```python
from build123d import *

# Parameters (mm, degrees)
BOSS_EXTRUDE1_DEPTH     = 3.175
SKETCH2_R               = 6.35
CUT_EXTRUDE1_DEPTH      = 4.1750001
CUT_EXTRUDE2_DEPTH      = 13.851031146
CUT_EXTRUDE2_DEPTH_BACK = 13.851031146


with BuildPart() as part:
    # Sketch1 → Boss-Extrude1 (new body)
    with BuildSketch(Plane.XY):
        with BuildLine():
            add(Edge.make_bspline(
                [(214.122, 0.26979372), (214.042517561, 0.336401081), (213.528971009, 0.273510814), (212.614475706, 0.530942112), (210.937412976, 0.69005818), (208.678154781, 1.031540783), (205.767891794, 1.412612557), (202.258298365, 1.882266), (198.158505405, 2.4131646), (193.498201346, 3.004251359), (188.3046229, 3.645171414), (182.610259265, 4.327250831), (176.450111776, 5.042029836), (169.862114854, 5.779776892), (162.886908752, 6.531484704), (155.567547263, 7.287816965), (147.949138879, 8.039011284), (140.078674392, 8.774523149), (132.004623532, 9.484696808), (123.776853773, 10.157659428), (115.445921162, 10.782438327), (107.063264355, 11.347433986), (98.680532246, 11.840832833), (90.349330839, 12.250169768), (82.121113367, 12.564529441), (74.046372156, 12.77365626), (66.175007458, 12.867335678), (58.555385553, 12.838133258), (51.234483397, 12.680408315), (44.257364483, 12.390162696), (37.666974317, 11.966637162), (31.503817676, 11.411106073), (25.805608692, 10.727908153), (20.607079774, 9.922856403), (15.939732749, 9.004358901), (11.830923582, 7.982801344), (8.304000309, 6.868145192), (5.376882013, 5.670771919), (3.058903356, 4.398782317), (1.353631156, 3.049665872), (0.261418186, 1.590784391), (-0.121830169, 0), (0.261418186, -1.590784391), (1.353631156, -3.049665872), (3.058903356, -4.398782317), (5.376882013, -5.670771919), (8.304000309, -6.868145192), (11.830923582, -7.982801344), (15.939732749, -9.004358901), (20.607079774, -9.922856403), (25.805608692, -10.727908153), (31.503817676, -11.411106073), (37.666974317, -11.966637162), (44.257364483, -12.390162696), (51.234483397, -12.680408315), (58.555385553, -12.838133258), (66.175007458, -12.867335678), (74.046372156, -12.77365626), (82.121113367, -12.564529441), (90.349330839, -12.250169768), (98.680532246, -11.840832833), (107.063264355, -11.347433986), (115.445921162, -10.782438327), (123.776853773, -10.157659428), (132.004623532, -9.484696808), (140.078674392, -8.774523149), (147.949138879, -8.039011284), (155.567547263, -7.287816965), (162.886908752, -6.531484704), (169.862114854, -5.779776892), (176.450111776, -5.042029836), (182.610259265, -4.327250831), (188.3046229, -3.645171414), (193.498201346, -3.004251359), (198.158505405, -2.4131646), (202.258298365, -1.882266), (205.767891794, -1.412612557), (208.678154781, -1.031540783), (210.937412976, -0.69005818), (212.614475706, -0.530942112), (213.528971009, -0.273510814), (214.25071943, -0.361898032), (214.25071943, 0.161925093), (214.122, 0.26979372)],
                knots=[0, 0, 0, 0, 0.000762215, 0.003044706, 0.006832246, 0.012101176, 0.018817536, 0.026939455, 0.036414848, 0.047184629, 0.059180413, 0.072327874, 0.086544061, 0.10174058, 0.117823336, 0.134691452, 0.152240154, 0.17036129, 0.188941008, 0.207865435, 0.227016078, 0.246275696, 0.265524943, 0.284644966, 0.303520118, 0.322034575, 0.340078353, 0.357542593, 0.374325482, 0.390329891, 0.40546389, 0.419643801, 0.432793371, 0.444843817, 0.455737921, 0.465428653, 0.47388632, 0.481101634, 0.487101684, 0.491975368, 0.495930678, 0.499382808, 0.502834938, 0.506790248, 0.511663932, 0.517663982, 0.524879296, 0.533336963, 0.543027695, 0.553921799, 0.565972245, 0.579121815, 0.593301726, 0.608435725, 0.624440134, 0.641223023, 0.658687263, 0.676731041, 0.695245498, 0.71412065, 0.733240673, 0.75248992, 0.771749538, 0.790900181, 0.809824608, 0.828404326, 0.846525462, 0.864074164, 0.88094228, 0.897025036, 0.912221555, 0.926437743, 0.939585203, 0.951580988, 0.962350768, 0.971826161, 0.979948081, 0.98666444, 0.991933371, 0.99572091, 0.998003402, 0.998765616, 1, 1, 1, 1], degree=3))
        make_face()
    extrude(amount=BOSS_EXTRUDE1_DEPTH)

    # Sketch2 → Cut-Extrude1 (cut, through all)
    with BuildSketch(Plane.XY.offset(3.175)):
        with Locations((25.4, 0)):
            Circle(SKETCH2_R)
        with Locations((101.6, 0)):
            Circle(SKETCH2_R)
    extrude(amount=-CUT_EXTRUDE1_DEPTH, mode=Mode.SUBTRACT)

    # Sketch4 → Cut-Extrude2 (cut, two sides)
    with BuildSketch(Plane(origin=(0, 0, 0), x_dir=(1, 0, 0), z_dir=(0, 1, 0))) as cut_extrude2_sk:
        Polygon((131.301372669, 0), (130.854723983, -3.175), (214.218539573, -3.175), (214.218539573, 0), align=None)
    extrude(amount=CUT_EXTRUDE2_DEPTH, mode=Mode.SUBTRACT)
    extrude(cut_extrude2_sk.sketch, amount=-CUT_EXTRUDE2_DEPTH_BACK, mode=Mode.SUBTRACT)

    # Sketch6 → Cut-Loft1 section 0
    with BuildSketch(Plane.XY.offset(3.175)):
        with BuildLine():
            Line((19.05, -5.856388973), (19.05, -9.60451625))
            Line((19.05, -9.60451625), (19.05, -13.496705478))
            Line((19.05, -13.496705478), (-3.17679028, -18.7418168))
            Line((-3.17679028, -18.7418168), (-7.400210772, 8.670878009))
            Line((-7.400210772, 8.670878009), (19.05, 13.499844305))
            Line((19.05, 13.499844305), (19.05, 9.60451625))
            Line((19.05, 9.60451625), (19.05, 5.856388972))
            Line((19.05, 5.856388972), (16.002, 5.855689085))
            add(Edge.make_bspline(
                [(16.002, 5.855689085), (15.278985699, 5.689672728), (14.191834186, 5.424851558), (12.757843363, 5.037907465), (11.69367278, 4.729775055), (10.646700316, 4.403337894), (9.617692504, 4.055796047), (8.608301637, 3.684577658), (7.626216232, 3.28790719), (6.678573411, 2.8637313), (5.779182107, 2.40890834), (5.078910801, 2.000461241), (4.5709467, 1.665455737), (4.220151013, 1.411514439), (3.905914023, 1.157647081), (3.631157505, 0.904651906), (3.399885574, 0.653944439), (3.226743451, 0.433066972), (3.126676284, 0.2697322), (3.07552602, 0.144421915), (3.049218429, 0.037663177), (3.047390298, 5.5e-08), (3.04921854, -0.03766331), (3.075525744, -0.1444217), (3.126676947, -0.269732641), (3.226742145, -0.433066135), (3.399888053, -0.653946015), (3.631152817, -0.904648933), (3.905923107, -1.157652839), (4.220131475, -1.411502059), (4.570981553, -1.665477812), (5.078773369, -2.000374258), (5.77925724, -2.408956031), (6.678536824, -2.863707828), (7.626233895, -3.287919031), (8.608295197, -3.684572243), (9.617690306, -4.05579733), (10.64671253, -4.403340225), (11.693641898, -4.729767367), (12.757897505, -5.037921267), (14.191640812, -5.424801637), (15.278985699, -5.689672728), (16.002, -5.855689085)],
                knots=[0, 0, 0, 0, 0.0625, 0.09375, 0.125, 0.15625, 0.1875, 0.21875, 0.25, 0.28125, 0.3125, 0.34375, 0.359375, 0.375, 0.390625, 0.40625, 0.421875, 0.4375, 0.453125, 0.46875, 0.484375, 0.5, 0.515625, 0.53125, 0.546875, 0.5625, 0.578125, 0.59375, 0.609375, 0.625, 0.640625, 0.65625, 0.6875, 0.71875, 0.75, 0.78125, 0.8125, 0.84375, 0.875, 0.90625, 0.9375, 1, 1, 1, 1], degree=3))
            Line((16.002, -5.855689085), (19.05, -5.856388973))
        make_face()
    # Sketch5 → Cut-Loft1 section 1
    with BuildSketch(Plane(origin=(0, 0, 0), x_dir=(-1, 0, 0), z_dir=(0, 0, -1))):
        with BuildLine():
            Line((-19.05, -9.69489598), (-19.05, -5.952242124))
            Line((-19.05, -5.952242124), (-16.002, -5.952242124))
            add(Edge.make_bspline(
                [(-16.002, 5.952242124), (-15.254770655, 5.78657596), (-14.131320952, 5.521981031), (-12.64893123, 5.134599211), (-11.548436123, 4.825723352), (-10.465051878, 4.498073941), (-9.399590771, 4.148800211), (-8.353696965, 3.775270971), (-7.504851445, 3.442218555), (-6.842934482, 3.161623807), (-6.194794877, 2.871042337), (-5.414728041, 2.488039147), (-4.683877816, 2.074629942), (-4.151373193, 1.734752799), (-3.782164679, 1.476616997), (-3.449549124, 1.21792525), (-3.156545696, 0.959314296), (-2.90735717, 0.702084345), (-2.716911913, 0.473376027), (-2.620007494, 0.329250424), (-2.568278365, 0.232230216), (-2.539730887, 0.166366119), (-2.518563335, 0.105023254), (-2.505407276, 0.055343345), (-2.499698937, 0.022962059), (-2.498722808, 3.7e-08), (-2.499699014, -0.022962102), (-2.505407277, -0.055343359), (-2.518563346, -0.105023288), (-2.539730598, -0.166365891), (-2.568278462, -0.232230258), (-2.620012631, -0.329254292), (-2.716907842, -0.47337309), (-2.907361053, -0.702086989), (-3.156540251, -0.959310743), (-3.449558648, -1.217931354), (-3.782145051, -1.476604524), (-4.151407833, -1.734774759), (-4.683741695, -2.074543768), (-5.414804155, -2.48808676), (-6.194777113, -2.871030834), (-6.84292503, -3.16161805), (-7.50486635, -3.442227642), (-8.353689563, -3.77526546), (-9.399589141, -4.148801556), (-10.465063669, -4.498076208), (-11.54840573, -4.825715767), (-12.648984703, -5.134612855), (-14.131129756, -5.52193166), (-15.254770655, -5.78657596), (-16.002, -5.952242124)],
                knots=[0, 0, 0, 0, 0.0625, 0.09375, 0.125, 0.15625, 0.1875, 0.21875, 0.25, 0.265625, 0.28125, 0.3125, 0.34375, 0.359375, 0.375, 0.390625, 0.40625, 0.421875, 0.4375, 0.453125, 0.4609375, 0.46875, 0.4765625, 0.484375, 0.4921875, 0.5, 0.5078125, 0.515625, 0.5234375, 0.53125, 0.5390625, 0.546875, 0.5625, 0.578125, 0.59375, 0.609375, 0.625, 0.640625, 0.65625, 0.6875, 0.71875, 0.734375, 0.75, 0.78125, 0.8125, 0.84375, 0.875, 0.90625, 0.9375, 1, 1, 1, 1], degree=3))
            Line((-16.002, 5.952242124), (-19.05, 5.952242124))
            Line((-19.05, 5.952242124), (-19.05, 9.69489598))
            Line((-19.05, 9.69489598), (-19.05, 12.377646409))
            Line((-19.05, 12.377646409), (3.93721866, 8.635694366))
            Line((3.93721866, 8.635694366), (2.51171312, -11.744580154))
            Line((2.51171312, -11.744580154), (-19.05, -12.301418255))
            Line((-19.05, -12.301418255), (-19.05, -9.69489598))
        make_face()
    loft(mode=Mode.SUBTRACT)


solid = part.part
```
Could you check a few things on this model? Use its own coordinates, in mm. Give positions to 0.01 mm unless a question says otherwise; leave off trailing zeros. One line per item, written item: value. Start each with the question number.
Item 1: Imagine slicing it at A-A, the plane y = 0. Give the number of separate pieces and of enclosed holes in the cut face, and give its area (3 significant figures).
Item 2: I'm going to push flat-ended pins straight in: pin 1 (10 mm diameter, centred on x = 25.4, y = 0, fed in from +Z); pin 2 (12 mm diameter, centred on x = 77, y = -8, fed in from -Z); pin 3 (1.5 mm diameter, centred on y = -4, z = 2.5, fed in from -X). Where does each tip first touch, or does it pass through?
Item 3: If we mould it in two halves opening along X, with no side actions, what happens to faces 1 (the face through (131.08, -0.13, 1.57)), 2 (the face through (107.657, 1.907, 1.61)), 3 (the face through (66, 0, 0))? For each: +X half, -X half, draft (parallel to the pull), parting line (faces both ways), or undercut.
Item 4: Please list where these lines run through material, in increasing order: line 1 (X direction, y = 2.25, z = 0.6); line 2 (Y direction, x = 101.6, z = 1.5); line 3 (Y direction, x = 21, z = 0.3). Write a range as from..to.
Geometry says:
1. separate pieces: 3
1. enclosed holes: 0
1. area: 327 mm^2
2. pin 1: through
2. pin 2: z = 0
2. pin 3: x = 7.44
3. face 1: +X half
3. face 2: undercut
3. face 3: draft
4. line 1: 5.1..19.46, 31.34..95.66, 107.54..131.22
4. line 2: -11.66..-6.35, 6.35..11.66
4. line 3: -9.96..-4.58, 4.58..9.96
